from build123d import *
from build123d.topology import SkipClean

# Parameters (mm, degrees)
SKETCH2_R                = 17.199960221
SKETCH2_R_2              = 12.422193493
SKETCH2_R_3              = 8.504424776
BOSS_EXTRUDE2_DEPTH      = 52
SKETCH4_R                = 13
CUT_EXTRUDE1_DEPTH       = 13
CUT_EXTRUDE2_START       = -13
SKETCH5_R                = 13
CUT_EXTRUDE2_DEPTH       = 13
SKETCH6_R                = 8.9
CUT_EXTRUDE3_DEPTH       = 59.45373069
CUT_EXTRUDE4_DEPTH       = 5
CUT_EXTRUDE5_START       = -5
CUT_EXTRUDE5_DEPTH       = 5
CUT_EXTRUDE6_START       = -2.25
CUT_EXTRUDE6_DEPTH       = 2.25
CUT_EXTRUDE7_DEPTH       = 2.25
CUT_EXTRUDE9_START       = -5.75
CUT_EXTRUDE9_DEPTH       = 5.75
CUT_EXTRUDE10_DEPTH      = 5.75
BOSS_EXTRUDE3_DEPTH      = 0.01
BOSS_EXTRUDE3_DEPTH_BACK = 10
SKETCH13_R               = 17.199960221
BOSS_EXTRUDE4_DEPTH      = 0.01
BOSS_EXTRUDE4_DEPTH_BACK = 10
SKETCH15_R               = 17.199960221
SKETCH16_R               = 17
CUT_EXTRUDE11_DEPTH      = 10
SKETCH17_R               = 9
CUT_EXTRUDE12_DEPTH      = 40
CHAMFER3_SIZE            = 1
CHAMFER3_SIZE_2          = 1.732050808


with BuildPart() as part:
    # Sketch2 → Boss-Extrude2 (new body)
    # profile 1 of 3: a face of its own
    with BuildSketch(Plane.XY):
        with BuildLine():
            Line((17.199960221, 40), (-17.199960221, 40))
            Line((-17.199960221, 40), (-17.199960221, 0))
            ThreePointArc((-17.199960221, 0), (0, 17.199960221), (17.199960221, 0))
            Line((17.199960221, 0), (17.199960221, 40))
        make_face()
    # profile 2 of 3: a face of its own
    with BuildSketch(Plane.XY):
        Circle(SKETCH2_R)
        Circle(SKETCH2_R_2, mode=Mode.SUBTRACT)
    # profile 3 of 3: a face of its own
    with BuildSketch(Plane.XY):
        Circle(SKETCH2_R_2)
        with Locations(Location((0, 0, 0), (0, 0, 180))):
            Circle(SKETCH2_R_3, mode=Mode.SUBTRACT)
    extrude(amount=BOSS_EXTRUDE2_DEPTH)

    # Sketch4 → Cut-Extrude1 (cut)
    with BuildSketch(Plane(origin=(0, 0, 0), x_dir=(-1, 0, 0), z_dir=(0, 0, -1))):
        Circle(SKETCH4_R)
    extrude(amount=-CUT_EXTRUDE1_DEPTH, mode=Mode.SUBTRACT)

    # Sketch5 → Cut-Extrude2 (cut)
    with BuildSketch(Plane.XY.offset(52).offset(CUT_EXTRUDE2_START)):
        with Locations(Location((0, 0, 0), (0, 0, 180))):
            Circle(SKETCH5_R)
    extrude(amount=CUT_EXTRUDE2_DEPTH, mode=Mode.SUBTRACT)

    # Sketch6 → Cut-Extrude3 (cut, through all)
    with BuildSketch(Plane.XY.offset(39)):
        Circle(SKETCH6_R)
    extrude(amount=-CUT_EXTRUDE3_DEPTH, mode=Mode.SUBTRACT)

    # Sketch7 → Cut-Extrude4 (cut)
    with BuildSketch(Plane(origin=(0, 0, 0), x_dir=(-1, 0, 0), z_dir=(0, 0, -1))):
        with BuildLine():
            Line((-17.199960221, 0), (-17.199960221, 40))
            Line((-17.199960221, 40), (17.199960221, 40))
            Line((17.199960221, 40), (17.199960221, 0))
            ThreePointArc((17.199960221, 0), (0, 17.199960221), (-17.199960221, 0))
        make_face()
    extrude(amount=-CUT_EXTRUDE4_DEPTH, mode=Mode.SUBTRACT)

    # Sketch8 → Cut-Extrude5 (cut)
    with BuildSketch(Plane.XY.offset(52).offset(CUT_EXTRUDE5_START)):
        with BuildLine():
            Line((-17.199960221, 0), (-17.199960221, 40))
            Line((-17.199960221, 40), (17.199960221, 40))
            Line((17.199960221, 40), (17.199960221, 0))
            ThreePointArc((17.199960221, 0), (0, 17.199960221), (-17.199960221, 0))
        make_face()
    extrude(amount=CUT_EXTRUDE5_DEPTH, mode=Mode.SUBTRACT)

    # Sketch9 → Cut-Extrude6 (cut)
    with BuildSketch(Plane.XY.offset(47).offset(CUT_EXTRUDE6_START)):
        with BuildLine():
            Line((-17.199960221, 37), (17.199960221, 37))
            Line((17.199960221, 37), (17.199960221, 0))
            ThreePointArc((17.199960221, 0), (0, 17.199960221), (-17.199960221, 0))
            Line((-17.199960221, 0), (-17.199960221, 37))
        make_face()
    extrude(amount=CUT_EXTRUDE6_DEPTH, mode=Mode.SUBTRACT)

    # Sketch10 → Cut-Extrude7 (cut)
    with SkipClean():  # the faces are left unmerged after this step: merging them gives an invalid solid
        with BuildSketch(Plane(origin=(0, 0, 5), x_dir=(-1, 0, 0), z_dir=(0, 0, -1))):
            with BuildLine():
                Line((-17.199960221, 37), (17.199960221, 37))
                Line((17.199960221, 37), (17.199960221, 0))
                ThreePointArc((17.199960221, 0), (0, 17.199960221), (-17.199960221, 0))
                Line((-17.199960221, 0), (-17.199960221, 37))
            make_face()
        extrude(amount=-CUT_EXTRUDE7_DEPTH, mode=Mode.SUBTRACT)
    add(part.part.scale(1), mode=Mode.REPLACE)  # the faces are merged on a copy

    # Sketch11 → Cut-Extrude9 (cut)
    with BuildSketch(Plane.XY.offset(44.75).offset(CUT_EXTRUDE9_START)):
        with BuildLine():
            Line((-17.199960221, 27), (17.199960221, 27))
            Line((17.199960221, 27), (17.199960221, 0))
            ThreePointArc((17.199960221, 0), (0, 17.199960221), (-17.199960221, 0))
            Line((-17.199960221, 0), (-17.199960221, 27))
        make_face()
    extrude(amount=CUT_EXTRUDE9_DEPTH, mode=Mode.SUBTRACT)

    # Sketch12 → Cut-Extrude10 (cut)
    with BuildSketch(Plane(origin=(0, 0, 7.25), x_dir=(-1, 0, 0), z_dir=(0, 0, -1))):
        with BuildLine():
            Line((-17.199960221, 27), (17.199960221, 27))
            Line((17.199960221, 27), (17.199960221, 0))
            ThreePointArc((17.199960221, 0), (0, 17.199960221), (-17.199960221, 0))
            Line((-17.199960221, 0), (-17.199960221, 27))
        make_face()
    extrude(amount=-CUT_EXTRUDE10_DEPTH, mode=Mode.SUBTRACT)

    # Sketch13 → Boss-Extrude3 (add, two sides: drawn at the far end of the back side and taken through both)
    with BuildSketch(Plane(origin=(0, 0, 0), x_dir=(-1, 0, 0), z_dir=(0, 0, -1)).offset(-BOSS_EXTRUDE3_DEPTH_BACK)):
        Polygon((-0.103617408, -20.784351408), (17.947967616, -10.481911012), (18.051585024, 10.302440396), (0.103617408, 20.784351408), (0, 20.725214652), (-17.947967616, 10.481911012), (-18.051585024, -10.302440396), align=None)
        Circle(SKETCH13_R, mode=Mode.SUBTRACT)
    extrude(amount=BOSS_EXTRUDE3_DEPTH + BOSS_EXTRUDE3_DEPTH_BACK)

    # Sketch15 → Boss-Extrude4 (add, two sides: drawn at the far end of the back side and taken through both)
    with BuildSketch(Plane.XY.offset(52).offset(-BOSS_EXTRUDE4_DEPTH_BACK)):
        Polygon((-18.051585024, 10.302440396), (-17.947967616, -10.481911012), (0.103617408, -20.784351408), (18.051585024, -10.302440396), (17.947967616, 10.481911012), (-0.103617408, 20.784351408), align=None)
        with Locations(Location((0, 0, 0), (0, 0, 180))):
            Circle(SKETCH15_R, mode=Mode.SUBTRACT)
    extrude(amount=BOSS_EXTRUDE4_DEPTH + BOSS_EXTRUDE4_DEPTH_BACK)

    # Sketch16 → Cut-Extrude11 (cut)
    with BuildSketch(Plane(origin=(0, 40, 0), x_dir=(1, 0, 0), z_dir=(0, 1, 0))):
        with Locations(Location((0, -26, 0), (0, 0, 270))):
            Circle(SKETCH16_R)
    extrude(amount=-CUT_EXTRUDE11_DEPTH, mode=Mode.SUBTRACT)

    # Sketch17 → Cut-Extrude12 (cut)
    with BuildSketch(Plane(origin=(0, 30, 0), x_dir=(1, 0, 0), z_dir=(0, 1, 0))):
        with Locations(Location((0, -26, 0), (0, 0, 270))):
            Circle(SKETCH17_R)
    extrude(amount=-CUT_EXTRUDE12_DEPTH, mode=Mode.SUBTRACT)

    # Chamfer3
    # the kernel refuses this chamfer: 1.732050808, 1 mm, written as the material it takes off along each edge
    with BuildSketch(Plane(origin=(21.92099597, -8.042640174, -0.01), x_dir=(0.029196521986656933, -0.04999262353370063, 0.9983227437537924), z_dir=(-0.8635219945420718, -0.5043111786804675, 0)), Plane(origin=(3.99536728, -23.005459473, -0.01), x_dir=(-0.028696620988686708, -0.050281241509443776, 0.9983227437537926), z_dir=(-0.8685072894207939, 0.4956763946598076, 0)), Plane(origin=(-17.925628689, -14.962819299, -0.01), x_dir=(-0.05789314297534289, -0.0002886179757454726, 0.9983227437537926), z_dir=(-0.004985294878722003, 0.9999875733402752, 0)), Plane(origin=(-21.92099597, 8.042640174, -0.01), x_dir=(-0.029196521986655326, 0.04999262353369786, 0.9983227437537926), z_dir=(0.8635219945420716, 0.5043111786804677, 0)), Plane(origin=(17.925628689, 14.962819299, -0.01), x_dir=(0.05789314297534289, 0.0002886179757454726, 0.9983227437537926), z_dir=(0.004985294878722003, -0.9999875733402752, 0)), Plane(origin=(-18.073923951, 14.783348683, 52.01), x_dir=(-0.05789314297534298, -0.00028861797574591844, -0.9983227437537926), z_dir=(0.004985294878729695, -0.9999875733402751, 0)), Plane(origin=(-21.839717488, -8.260802946, 52.01), x_dir=(-0.028696620988686607, -0.05028124150944443, -0.9983227437537926), z_dir=(0.8685072894207975, -0.49567639465980146, 0)), Plane(origin=(-3.765793537, -23.044151629, 52.01), x_dir=(0.02919652198665585, -0.04999262353369789, -0.9983227437537927), z_dir=(0.8635219945420678, 0.5043111786804741, 0)), Plane(origin=(18.073923951, -14.783348683, 52.01), x_dir=(0.057893142975342975, 0.00028861797574592825, -0.9983227437537926), z_dir=(-0.004985294878729864, 0.9999875733402751, 0)), Plane(origin=(21.839717488, 8.260802946, 52.01), x_dir=(0.02869662098868756, 0.050281241509446094, -0.9983227437537926), z_dir=(-0.8685072894207974, 0.4956763946598015, 0)), Plane(origin=(3.765793537, 23.044151629, 52.01), x_dir=(-0.029196521986655923, 0.04999262353369809, -0.9983227437537926), z_dir=(-0.8635219945420681, -0.5043111786804736, 0))) as chamfer3_piece_1:
        Polygon((CHAMFER3_SIZE * 0.998322743754, CHAMFER3_SIZE * 0.0578938624027), (-CHAMFER3_SIZE_2 * 0.0578938623883, CHAMFER3_SIZE_2 * 0.998322743505), (0, 0), align=None)
    extrude(amount=29.746537632, mode=Mode.SUBTRACT)
    with BuildSketch(Plane(origin=(21.839717488, 8.260802946, -0.01), x_dir=(0.02869662098868796, 0.05028124150944598, 0.9983227437537924), z_dir=(-0.8685072894207939, 0.4956763946598075, 0))) as chamfer3_piece_2:
        Polygon((CHAMFER3_SIZE * 0.998322743754, -CHAMFER3_SIZE * 0.0578938624027), (-CHAMFER3_SIZE_2 * 0.0578938623883, -CHAMFER3_SIZE_2 * 0.998322743505), (0, 0), align=None)
    extrude(amount=29.746537632, mode=Mode.SUBTRACT)


solid = part.part
Can you work these out from the model? Positions are in its coordinate system, mm. A direction names the side the tool comes from. Round coordinates to 2 decimals unless told otherwise and drop trailing zeros. Loops run counter-clockwise (first coordinate to the right, second up) from the corner with the lowest first, then second, coordinate; pieces in that order, holes last. Notation, with made-up numbers: (-15, 52) - (1, 52) arc R35 cw to (1, 87) - close; hole circle Ø9 at (33.25, 58). An arc over 180 degrees is marked (long way). Answer in a Markdown table with one row per item. Add a question column.
Q1. We'd pull the mould along Y, two halves only. Please class faces 1 (the flat face through (-6, 8, 39)), 2 (the flat face through (15, -9, -0.01)), 3 (the flat face through (0, -10, 26)), 4 (the flat face through (-9.2, 15.47, 5.56)): pulls with the +Y half, pulls with the -Y half, needs draft (parallel to the pull), parting line crosses it, or undercut.
Q2. I want a section at C-C on x = -7. Count the separate pieces of the cut face and the enclosed holes in it, and give its area (3 significant figures).
Q3. I want a section at B-B on y = 25.5. List the corners of the cut face in (x, z) for me, and give its area (3 significant figures).
Q4. For pin 1 Ø2 at (y, z) = (23, 44.5) entering from +X; pin 2 Ø2 at (x, y) = (5.5, -7.5) entering from -Z; pin 3 Ø21 at (x, y) = (2.5, 1.5) entering from -Z; pin 4 Ø2 at (y, z) = (32, 25) entering from +X, each with a flat end and sliding along its axis, tell me the tip position at first contact or that it passes through.
Q5. I want a section at D-D on z = 20.5. List the corners of the cut face in (x, y) for me.
Q6. Which directions (+Z, -Z, +X, -X, +Y, -Y) give clear straight access to the entire face, cutting with the end or side of a thin tool? Please do faces 5 (the flat face through (4, -17, 10)), 6 (the flat face through (-8.5, 14.9, 51.5)).
Q7. I need wall thicknesses on L1, parallel to X at y = 36, z = 26; L2, parallel to Y at x = -5, z = 45; L3, parallel to X at y = 0, z = 20. Which ranges of each line are inside material? Lowest first, please.
Q8. I want a section at A-A on z = 12. List the corners of the cut face in (x, y) for me, and give its area (3 significant figures).
A:
| question | item | result |
|---|---|---|
| 1 | face 1 | undercut |
| 1 | face 2 | needs draft |
| 1 | face 3 | pulls with the +Y half |
| 1 | face 4 | undercut |
| 2 | separate pieces | 3 |
| 2 | enclosed holes | 0 |
| 2 | area | 972 mm^2 |
| 3 | outline | (-17.2, 13) - (17.2, 13) - (17.2, 39) - (-17.2, 39) - close; hole circle Ø18 at (0, 26) |
| 3 | area | 640 mm^2 |
| 4 | pin 1 | through |
| 4 | pin 2 | z = 13 |
| 4 | pin 3 | z = 0 |
| 4 | pin 4 | x = 17.2 |
| 5 | outline | (-17.2, 0) arc R17.2 ccw to (17.2, 0) - (17.2, 40) - (16.09, 40) - (16.09, 30) - (7.12, 30) - (7.12, 5.33) arc R8.9 cw to (7.12, -5.33) - (7.12, -10) - (-7.12, -10) - (-7.12, -5.33) arc R8.9 cw to (-7.12, 5.33) - (-7.12, 30) - (-16.09, 30) - (-16.09, 40) - (-17.2, 40) - close |
| 6 | face 5 | none |
| 6 | face 6 | +Z, -X, +Y |
| 7 | L1 | -17.2 to -17, 17 to 17.2 |
| 7 | L2 | -17.87 to -12, 12 to 17.92, 37 to 40 |
| 7 | L3 | -17.2 to -8.9, 8.9 to 17.2 |
| 8 | outline | circle Ø34.4 at (0, 0); (-17.2, 27) - (17.2, 27) - (17.2, 40) - (9.64, 40) - (9.64, 30) - (-9.64, 30) - (-9.64, 40) - (-17.2, 40) - close; hole circle Ø26 at (0, 0) |
| 8 | area | 653 mm^2 |
